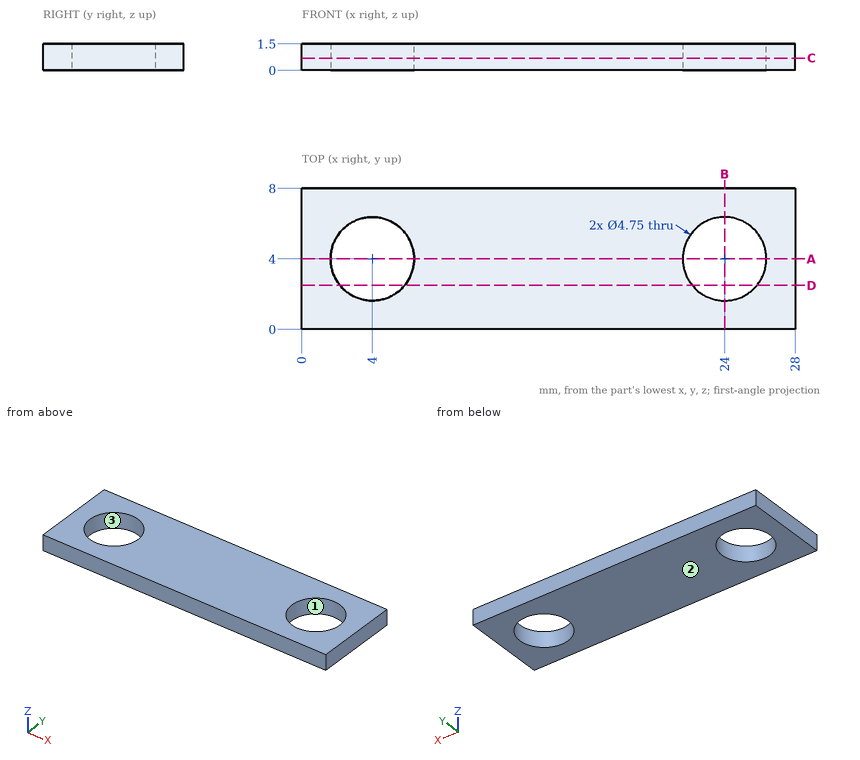
Geometry check sheet. Reference: drawing and pictorial views, mm from the part's lowest x, y, z. Give positions to 0.01 mm unless a question says otherwise; leave off trailing zeros. Loops run counter-clockwise (first coordinate to the right, second up) from the corner with the lowest first, then second, coordinate; pieces in that order, holes last. Notation, with made-up numbers: (-5, -24) - (-1, -24) arc R14 ccw to (-1, -8) - close; hole circle Ø8 at (16, 85). An arc over 180 degrees is marked (long way). One line per question, with ' | ' between items. Start each with the question number.
1. Material ranges on line 1 along Y through (x, z) = (24, 1.1) (3 decimals); line 2 along X through (y, z) = (4.75, 0.95); line 3 along X through (y, z) = (3, 0.5), recorded low to high. Write a range as [from, to].
2. Cross-section at C-C, the plane z = 0.7. Enter the section's corners in (x, y) (3 decimals), plus the area to 3 significant figures.
3. Cross-section at D-D, the plane y = 2.5. Enter the section's corners in (x, z), plus the area to 3 significant figures.
4. Cross-section at A-A, the plane y = 4. Enter the section's corners in (x, z) (3 decimals), plus the area to 4 significant figures.
5. Draft check along Y on the marked faces 1, 2 and 3. Enter one of: released by +Y, released by -Y, zero draft, split by the parting line, or undercut.
6. Cross-section at B-B, the plane x = 24. Enter the section's corners in (y, z) (3 decimals), plus the area to 4 significant figures.
Check result:
1) line 1: y = [0, 1.625], [6.375, 8] | line 2: x = [0, 1.75], [6.25, 21.75], [26.25, 28] | line 3: x = [0, 1.85], [6.15, 21.85], [26.15, 28]
2) outline: (0, 0) - (28, 0) - (28, 8) - (0, 8) - close; hole circle Ø4.75 at (4, 4); hole circle Ø4.75 at (24, 4) | area: 189 mm2
3) outline: (0, 0) - (2.16, 0) - (2.16, 1.5) - (0, 1.5) - close; (5.84, 0) - (22.16, 0) - (22.16, 1.5) - (5.84, 1.5) - close; (25.84, 0) - (28, 0) - (28, 1.5) - (25.84, 1.5) - close | area: 31.0 mm2
4) outline: (0, 0) - (1.625, 0) - (1.625, 1.5) - (0, 1.5) - close; (6.375, 0) - (21.625, 0) - (21.625, 1.5) - (6.375, 1.5) - close; (26.375, 0) - (28, 0) - (28, 1.5) - (26.375, 1.5) - close | area: 27.75 mm2
5) face 1: undercut | face 2: zero draft | face 3: undercut
6) outline: (0, 0) - (1.625, 0) - (1.625, 1.5) - (0, 1.5) - close; (6.375, 0) - (8, 0) - (8, 1.5) - (6.375, 1.5) - close | area: 4.875 mm2
